Could you check a few things on this model? Use its own coordinates, in mm. A direction names the side the tool comes from. Give positions to 0.01 mm unless a question says otherwise; leave off trailing zeros. Write each loop counter-clockwise with the first axis right and the second up, starting at its lowest first coordinate (ties: lowest second). Pieces come first, ordered by that corner, then holes. Notation, with made-up numbers: (55.5, 82) - (69.5, 82) arc R12 cw to (69.5, 86) - close; hole circle Ø11 at (-7, 89). An arc over 180 degrees is marked (long way). Answer in a Markdown table with one row per item.
from build123d import *

# Parameters (mm, degrees)
F0_W            = 170
F0_H            = 50
F0_R            = 11.5
F1_DEPTH        = 10
F2_R            = 3.25
F3_DEPTH        = 10.001
F4_R            = 15
F4_R_2          = 11.5
F5_DEPTH        = 3
F7_DEPTH        = 25
F8_T1_DEPTH     = 20.004828627
F8_T3_DEPTH     = 12.3229236974
F8_T5_DEPTH     = 6.1336823274
F9_T1_DEPTH     = 46
F9_T3_DEPTH     = 166
F9_T5_DEPTH     = 13
F9_T7_DEPTH     = 80.0390459698
F9_T9_DEPTH     = 80.0390459698
F9_S13_W        = 2
F9_S13_H        = 2
F9_T14_DEPTH    = 2
F9_S19_W        = 2
F9_S19_H        = 2
F9_T20_DEPTH    = 2
F9_S25_W        = 2
F9_S25_H        = 2
F9_T26_DEPTH    = 2
F9_S31_W        = 2
F9_S31_H        = 2
F9_T32_DEPTH    = 2
F11_D           = 6.5
F11_DEPTH       = 15
F11_CSINK_D     = 12
F11_CSINK_ANGLE = 90
F11_TIP         = 1.9527970118


# Not quite as in the source:
# - a fillet or chamfer that OpenCascade refuses, or shapes differently, is made with other operations: its cross-section is extruded or revolved along the edge and cut away or added


with BuildPart() as f1:
    # F0 (on Top) → F1 (new body)
    with BuildSketch(Plane.XY):
        Rectangle(F0_W, F0_H)
        Circle(F0_R, mode=Mode.SUBTRACT)
    extrude(amount=F1_DEPTH)

    # F2 (on face) → F3 (cut, through all)
    with BuildSketch(Plane.XY.offset(10)):
        with Locations((-75, 15)):
            Circle(F2_R)
        with Locations((-75, -15)):
            Circle(F2_R)
        with Locations((75, -15)):
            Circle(F2_R)
        with Locations((75, 15)):
            Circle(F2_R)
    extrude(amount=-F3_DEPTH, mode=Mode.SUBTRACT)

    # F4 (on face) → F5 (cut)
    with BuildSketch(Plane.XY.offset(10)):
        Circle(F4_R)
        Circle(F4_R_2, mode=Mode.SUBTRACT)
    extrude(amount=-F5_DEPTH, mode=Mode.SUBTRACT)

    # F6 (on face) → F7 (cut)
    with BuildSketch(Plane.XY.offset(10)):
        with BuildLine():
            Line((-6, -13.7477270849), (-6, -25))
            Line((-6, -25), (6, -25))
            Line((6, -25), (6, -13.7477270849))
            ThreePointArc((6, -13.7477270849), (0, -15), (-6, -13.7477270849))
        make_face()
        with BuildLine():
            Line((-6, -9), (-6, -13.7477270849))
            ThreePointArc((-6, -13.7477270849), (0, -15), (6, -13.7477270849))
            Line((6, -13.7477270849), (6, -9))
            Line((6, -9), (-6, -9))
        make_face()
    extrude(amount=-F7_DEPTH, mode=Mode.SUBTRACT)

    # F8: fillet of radius 2 on 5 edges, made by hand

    # F8_s2 → F8_t1 (cut)
    with BuildSketch(Plane.XY.offset(-5.0024143135)):
        with BuildLine():
            ThreePointArc((-5.9996, -22.9990343146), (-6.5857864376, -24.4142135624), (-8.0009656854, -25.0004))
            Line((-8.0009656854, -25.0004), (-8.0009656854, -25.2005365685))
            ThreePointArc((-8.0009656854, -25.2005365685), (-7.0004828427, -25.2001365685), (-6, -25.2001365685))
            Line((-6, -25.2001365685), (-5.7998634315, -25))
            ThreePointArc((-5.7998634315, -25), (-5.7998634315, -23.9995171573), (-5.7994634315, -22.9990343146))
            Line((-5.7994634315, -22.9990343146), (-5.9996, -22.9990343146))
        make_face()
        with BuildLine():
            ThreePointArc((5.9996, -22.9990343146), (6.5857864376, -24.4142135624), (8.0009656854, -25.0004))
            Line((8.0009656854, -25.0004), (8.0009656854, -25.2005365685))
            ThreePointArc((8.0009656854, -25.2005365685), (7.0004828427, -25.2001365685), (6, -25.2001365685))
            Line((6, -25.2001365685), (5.7998634315, -25))
            ThreePointArc((5.7998634315, -25), (5.7998634315, -23.9995171573), (5.7994634315, -22.9990343146))
            Line((5.7994634315, -22.9990343146), (5.9996, -22.9990343146))
        make_face()
    extrude(amount=F8_T1_DEPTH, mode=Mode.SUBTRACT)

    # F8_s4 → F8_t3 (cut)
    with BuildSketch(Plane.XY.offset(-2.6614618487)):
        with BuildLine():
            ThreePointArc((-6.8152717523, -9.2624441214), (-6.215115784, -9.9716058978), (-5.9996, -10.8752930995))
            Line((-5.9996, -10.8752930995), (-5.79936, -10.8752930995))
            ThreePointArc((-5.79936, -10.8752930995), (-5.79976, -10.3430007673), (-5.79976, -9.8107084352))
            Line((-5.79976, -9.8107084352), (-5.8955269565, -9.6398826737))
            ThreePointArc((-5.8955269565, -9.6398826737), (-6.3019268651, -9.3792480426), (-6.6965989276, -9.1011592236))
            Line((-6.6965989276, -9.1011592236), (-6.8152717523, -9.2624441214))
        make_face()
        with BuildLine():
            ThreePointArc((5.9996, -10.8752930995), (6.215115784, -9.9716058978), (6.8152717523, -9.2624441214))
            Line((6.8152717523, -9.2624441214), (6.6965989276, -9.1011592236))
            ThreePointArc((6.6965989276, -9.1011592236), (6.3019268651, -9.3792480426), (5.8955269565, -9.6398826737))
            Line((5.8955269565, -9.6398826737), (5.79976, -9.8107084352))
            ThreePointArc((5.79976, -9.8107084352), (5.79976, -10.3430007673), (5.79936, -10.8752930995))
            Line((5.79936, -10.8752930995), (5.9996, -10.8752930995))
        make_face()
    extrude(amount=F8_T3_DEPTH, mode=Mode.SUBTRACT)

    # F8_s6 → F8_t5 (cut)
    with BuildSketch(Plane.XY.offset(7)):
        with BuildLine():
            ThreePointArc((-7.0595694154, -13.2344429361), (-6.2849198093, -13.9710342475), (-5.9996, -15.001199952))
            Line((-5.9996, -15.001199952), (-5.79936, -15.001199952))
            ThreePointArc((-5.79936, -15.001199952), (-5.79976, -14.3744635184), (-5.79976, -13.7477270849))
            Line((-5.79976, -13.7477270849), (-5.919904, -13.5642040934))
            ThreePointArc((-5.919904, -13.5642040934), (-6.4476696186, -13.3214283223), (-6.9653263569, -13.0577672345))
            Line((-6.9653263569, -13.0577672345), (-7.0595694154, -13.2344429361))
        make_face()
    extrude(amount=F8_T5_DEPTH, mode=Mode.SUBTRACT)

    # F9: fillet of radius 2 on 9 edges, made by hand

    # F9_s2 → F9_t1 (cut)
    with BuildSketch(Plane.XZ.offset(-23)):
        with BuildLine():
            ThreePointArc((-83, 10), (-84.4142135624, 9.4142135624), (-85, 8))
            Line((-85, 8), (-85, 10))
            Line((-85, 10), (-83, 10))
        make_face()
        with BuildLine():
            ThreePointArc((85, 8), (84.4142135624, 9.4142135624), (83, 10))
            Line((83, 10), (85, 10))
            Line((85, 10), (85, 8))
        make_face()
    extrude(amount=F9_T1_DEPTH, mode=Mode.SUBTRACT)

    # F9_s4 → F9_t3 (cut)
    with BuildSketch(Plane.YZ.offset(-83)):
        with BuildLine():
            ThreePointArc((23, 10), (24.4142135624, 9.4142135624), (25, 8))
            Line((25, 8), (25, 10))
            Line((25, 10), (23, 10))
        make_face()
    extrude(amount=F9_T3_DEPTH, mode=Mode.SUBTRACT)

    # F9_s6 → F9_t5 (cut)
    with BuildSketch(Plane.XY.offset(-5)):
        with BuildLine():
            ThreePointArc((85, -23), (84.4142135624, -24.4142135624), (83, -25))
            Line((83, -25), (85, -25))
            Line((85, -25), (85, -23))
        make_face()
        with BuildLine():
            ThreePointArc((85, 23), (84.4142135624, 24.4142135624), (83, 25))
            Line((83, 25), (85, 25))
            Line((85, 25), (85, 23))
        make_face()
        with BuildLine():
            ThreePointArc((-85, -23), (-84.4142135624, -24.4142135624), (-83, -25))
            Line((-83, -25), (-85, -25))
            Line((-85, -25), (-85, -23))
        make_face()
        with BuildLine():
            ThreePointArc((-85, 23), (-84.4142135624, 24.4142135624), (-83, 25))
            Line((-83, 25), (-85, 25))
            Line((-85, 25), (-85, 23))
        make_face()
    extrude(amount=F9_T5_DEPTH, mode=Mode.SUBTRACT)

    # F9_s8 → F9_t7 (cut)
    with BuildSketch(Plane.YZ.offset(2.9609540302)):
        with BuildLine():
            ThreePointArc((-23, 10), (-24.4142135624, 9.4142135624), (-25, 8))
            Line((-25, 8), (-25, 10))
            Line((-25, 10), (-23, 10))
        make_face()
    extrude(amount=F9_T7_DEPTH, mode=Mode.SUBTRACT)

    # F9_s10 → F9_t9 (cut)
    with BuildSketch(Plane.YZ.offset(-83)):
        with BuildLine():
            ThreePointArc((-23, 10), (-24.4142135624, 9.4142135624), (-25, 8))
            Line((-25, 8), (-25, 10))
            Line((-25, 10), (-23, 10))
        make_face()
    extrude(amount=F9_T9_DEPTH, mode=Mode.SUBTRACT)


with BuildPart() as f9_tool12:
    # F9_s13 → F9_t14 (new body)
    with BuildSketch(Plane.XY.offset(8)):
        with Locations((-84, 24)):
            Rectangle(F9_S13_W, F9_S13_H)
    extrude(amount=F9_T14_DEPTH)

    # F9_s15 → F9_t16 (revolve, cut)
    with BuildSketch(Plane(origin=(-83, 23, 8), x_dir=(0.7071067812, -0.7071067812, 0), z_dir=(-0.7071067812, -0.7071067812, 0))):
        with BuildLine():
            ThreePointArc((0, -2), (2, 0), (0, 2))
            Line((0, 2), (0, -2))
        make_face()
    revolve(axis=Axis((-83, 23, 8), (0, 0, 1)), mode=Mode.SUBTRACT)


with BuildPart() as f1_1:
    add(f1.part)

    # F9_t11: cut F9_tool12
    add(f9_tool12.part, mode=Mode.SUBTRACT)


with BuildPart() as f9_tool18:
    # F9_s19 → F9_t20 (new body)
    with BuildSketch(Plane.XY.offset(8)):
        with Locations((-84, -24)):
            Rectangle(F9_S19_W, F9_S19_H)
    extrude(amount=F9_T20_DEPTH)

    # F9_s21 → F9_t22 (revolve, cut)
    with BuildSketch(Plane(origin=(-83, -23, 8), x_dir=(0.7071067812, 0.7071067812, 0), z_dir=(0.7071067812, -0.7071067812, 0))):
        with BuildLine():
            ThreePointArc((0, -2), (2, 0), (0, 2))
            Line((0, 2), (0, -2))
        make_face()
    revolve(axis=Axis((-83, -23, 8), (0, 0, 1)), mode=Mode.SUBTRACT)


with BuildPart() as f1_2:
    add(f1_1.part)

    # F9_t17: cut F9_tool18
    add(f9_tool18.part, mode=Mode.SUBTRACT)


with BuildPart() as f9_tool24:
    # F9_s25 → F9_t26 (new body)
    with BuildSketch(Plane.YZ.offset(83)):
        with Locations((24, 9)):
            Rectangle(F9_S25_W, F9_S25_H)
    extrude(amount=F9_T26_DEPTH)

    # F9_s27 → F9_t28 (revolve, cut)
    with BuildSketch(Plane(origin=(83, 23, 8), x_dir=(0, -0.7071067812, -0.7071067812), z_dir=(0, -0.7071067812, 0.7071067812))):
        with BuildLine():
            ThreePointArc((0, -2), (2, 0), (0, 2))
            Line((0, 2), (0, -2))
        make_face()
    revolve(axis=Axis((83, 23, 8), (1, 0, 0)), mode=Mode.SUBTRACT)


with BuildPart() as f1_3:
    add(f1_2.part)

    # F9_t23: cut F9_tool24
    add(f9_tool24.part, mode=Mode.SUBTRACT)


with BuildPart() as f9_tool30:
    # F9_s31 → F9_t32 (new body)
    with BuildSketch(Plane.YZ.offset(83)):
        with Locations((-24, 9)):
            Rectangle(F9_S31_W, F9_S31_H)
    extrude(amount=F9_T32_DEPTH)

    # F9_s33 → F9_t34 (revolve, cut)
    with BuildSketch(Plane(origin=(83, -23, 8), x_dir=(0, 0.7071067812, -0.7071067812), z_dir=(0, -0.7071067812, -0.7071067812))):
        with BuildLine():
            ThreePointArc((0, -2), (2, 0), (0, 2))
            Line((0, 2), (0, -2))
        make_face()
    revolve(axis=Axis((83, -23, 8), (1, 0, 0)), mode=Mode.SUBTRACT)


with BuildPart() as f1_4:
    add(f1_3.part)

    # F9_t29: cut F9_tool30
    add(f9_tool30.part, mode=Mode.SUBTRACT)

    # F11
    with Locations(Plane.XY.offset(10)):
        with Locations((-75, 15), (-75, -15), (75, -15), (75, 15)):
            CounterSinkHole(F11_D / 2, F11_CSINK_D / 2, depth=F11_DEPTH, counter_sink_angle=F11_CSINK_ANGLE)
            with Locations((0, 0, -(F11_DEPTH + F11_TIP / 2))):  # 118° drill point
                Cone(0, F11_D / 2, F11_TIP, mode=Mode.SUBTRACT)


solid = f1_4.part
1) Imagine slicing it at C-C (z = 5.25). List the corners of the cut face in (x, y) for me.
Check values:
| item | result |
|---|---|
| outline | (-85, -23) arc R2 ccw to (-83, -25) - (-7.96, -25) arc R2 ccw to (-6, -23.04) - (-6, -10.84) arc R2 ccw to (-6.79, -9.28) arc R11.5 cw (long way) to (6.79, -9.28) arc R2 ccw to (6, -10.84) - (6, -23.04) arc R2 ccw to (7.96, -25) - (83, -25) arc R2 ccw to (85, -23) - (85, 23) arc R2 ccw to (83, 25) - (-83, 25) arc R2 ccw to (-85, 23) - close; hole circle Ø6.5 at (-75, -15); hole circle Ø6.5 at (-75, 15); hole circle Ø6.5 at (75, -15); hole circle Ø6.5 at (75, 15) |
2) Will these pins go through, and if not, where does the flat tip stop? P1, Ø10.5, axis at x = -75, y = -15, coming from the +Z side; P2, Ø3, axis at y = -14.5, z = 9, coming from the +X side.
Check values:
| item | result |
|---|---|
| P1 | stops at z = 9.25 |
| P2 | stops at x = 85 |
3) We'd pull the mould along X, two halves only. Please class faces 4 (the face through (6, -17, 5)), 5 (the face through (-1, 17, 0)), 6 (the face through (-85, 0, 4)): +X half, -X half, draft (parallel to the pull), parting line (faces both ways), or undercut.
Check values:
| item | result |
|---|---|
| face 4 | undercut |
| face 5 | draft |
| face 6 | -X half |
4) Imagine slicing it at A-A (x = -75). List the corners of the cut face in (y, z) for me, then the cut area to 3 significant figures.
Check values:
| item | result |
|---|---|
| outline | (-25, 0) - (-18.25, 0) - (-18.25, 7.25) - (-21, 10) - (-23, 10) arc R2 ccw to (-25, 8) - close; (-11.75, 0) - (11.75, 0) - (11.75, 7.25) - (9, 10) - (-9, 10) - (-11.75, 7.25) - close; (18.25, 0) - (25, 0) - (25, 8) arc R2 ccw to (23, 10) - (21, 10) - (18.25, 7.25) - close |
| area | 353 mm2 |
5) On a 3-axis mill with a long thin cutter (end or side, diameter ignored), from which of +Z, -Z, +X, -X, +Y, -Y can I reach the whole of each face in a straight line? I mean faces 1 (the face through (1.134, 14.957, 8.521)), 2 (the face through (-6, -17, 5)), 3 (the face through (71.753, -14.857, 3.676)). Say none if no direction works.
Check values:
| item | result |
|---|---|
| face 1 | +Z |
| face 2 | +Z, -Z, -Y |
| face 3 | +Z, -Z |
6) If I drill on line 1 (X direction, y = -15, z = 2.25); line 2 (Y direction, x = 75, z = 4.75); line 3 (X direction, y = -12, z = 8), over which ranges is the centre line in solid material (lowest first)?
Check values:
| item | result |
|---|---|
| line 1 | x = -85 to -78.25, -71.75 to -6, 6 to 71.75, 78.25 to 85 |
| line 2 | y = -25 to -18.25, -11.75 to 11.75, 18.25 to 25 |
| line 3 | x = -85 to -77.65, -72.35 to -9, 9 to 72.35, 77.65 to 85 |
7) Imagine slicing it at B-B (y = 0). List the corners of the cut face in (x, z) for me, then the cut area to 3 significant figures.
Check values:
| item | result |
|---|---|
| outline | (-85, 0) - (-11.5, 0) - (-11.5, 7) - (-15, 7) - (-15, 10) - (-83, 10) arc R2 ccw to (-85, 8) - close; (11.5, 0) - (85, 0) - (85, 8) arc R2 ccw to (83, 10) - (15, 10) - (15, 7) - (11.5, 7) - close |
| area | 1,450 mm2 |
8) Imagine slicing it at D-D (x = 0). List the corners of the cut face in (y, z) for me, then the cut area to 3 significant figures.
Check values:
| item | result |
|---|---|
| outline | (11.5, 0) - (25, 0) - (25, 8) arc R2 ccw to (23, 10) - (15, 10) - (15, 7) - (11.5, 7) - close |
| area | 124 mm2 |
